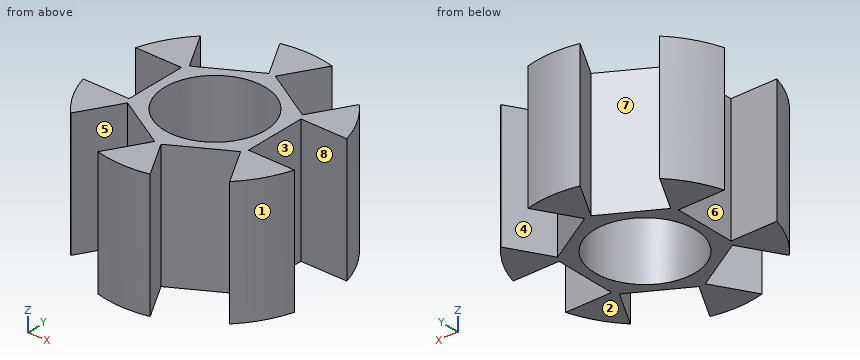
from build123d import *

# Parameters (mm, degrees)
SKETCH1_R           = 8.75
SKETCH1_R_2         = 4
BOSS_EXTRUDE1_DEPTH = 5
SKETCH2_W           = 4.9
SKETCH2_H           = 10
CUT_EXTRUDE3_DEPTH  = 4
CIRPATTERN1_COUNT   = 6


with BuildPart() as part:
    # Sketch1 → Boss-Extrude1 (new body, symmetric)
    with BuildSketch(Plane.XY):
        Circle(SKETCH1_R)
        Circle(SKETCH1_R_2, mode=Mode.SUBTRACT)
    extrude(amount=BOSS_EXTRUDE1_DEPTH, both=True)

    # Sketch2 → Cut-Extrude3 (cut)
    with BuildSketch(Plane(origin=(-8.75, -17.193061184, 0), x_dir=(0, -1, 0), z_dir=(1, 0, 0))):
        with Locations((-17.193061184, 0)):
            Rectangle(SKETCH2_W, SKETCH2_H)
    cut_extrude3 = extrude(amount=CUT_EXTRUDE3_DEPTH, mode=Mode.SUBTRACT)

    # CirPattern1: Cut-Extrude3 ×6 about axis
    cirpattern1_axis = Axis((0, 0, 0), (0, 0, 1))
    for i in range(1, CIRPATTERN1_COUNT):
        add(cut_extrude3.rotate(cirpattern1_axis, i * 360 / CIRPATTERN1_COUNT), mode=Mode.SUBTRACT)


solid = part.part
CAD build for the part. Positions are in the model's coordinates, mm. Face numbers are marked on the shaded views. A direction names the side the tool comes from. Give positions to 0.01 mm unless a question says otherwise; leave off trailing zeros. Write each loop counter-clockwise with the first axis right and the second up, starting at its lowest first coordinate (ties: lowest second). Pieces come first, ordered by that corner, then holes. Notation, with made-up numbers: (69, -35) - (92, -35) arc R20 cw to (92, -7) - close; hole circle Ø6 at (-13.75, 66). An arc over 180 degrees is marked (long way). Answer as CSV lines item,"result".
Q1. 3-axis set-ups, long thin cutter, end or side, ignore diameter. For the marked faces 4, 5, 6, 7 and 8: which of +Z, -Z, +X, -X, +Y, -Y reach the whole face in a straight line?
Result set:
face 4,"+Z, -Z, +Y"
face 5,"+Z, -Z, -Y"
face 6,"+Z, -Z, -X"
face 7,"+Z, -Z"
face 8,"+Z, -Z, +X"
Q2. Band-saw the part on D-D (x = -4.25). Give the cut face in (y, z), and give its area (3 significant figures).
Result set:
outline,"(-3.03, -5) - (3.03, -5) - (3.03, 5) - (-3.03, 5) - close"
area,"60.6 mm²"
Q3. Band-saw the part on A-A (x = 0). Give the cut face in (y, z).
Result set:
outline,"(-8.75, -5) - (-4, -5) - (-4, 5) - (-8.75, 5) - close; (4, -5) - (8.75, -5) - (8.75, 5) - (4, 5) - close"
Q4. Pull direction Y, two halves, no side cores. Call the marked faces 1, 2 and 3: released by +Y, released by -Y, zero draft, split by the parting line, or undercut.
Result set:
face 1,"released by -Y"
face 2,"zero draft"
face 3,"undercut"
Q5. Band-saw the part on B-B (y = 0). Give the cut face in (x, z).
Result set:
outline,"(-4.75, -5) - (-4, -5) - (-4, 5) - (-4.75, 5) - close; (4, -5) - (4.75, -5) - (4.75, 5) - (4, 5) - close"
Q6. Drill centre lines: line 1 (Y direction, x = 0, z = -2.5); line 2 (X direction, y = -4.5, z = 2.75); line 3 (Y direction, x = -0.5, z = 2.75). Where is each one in solid material? Low to high. Write a range as from..to.
Result set:
line 1,"-8.75..-4, 4..8.75"
line 2,"-7.5..-5.43, -1.71..1.71, 5.43..7.5"
line 3,"-8.74..-5.77, -5.2..-3.97, 3.97..5.2, 5.77..8.74"
Q7. Band-saw the part on C-C (z = 3.5). Give the cut face in (x, y), and give its area (3 significant figures).
Result set:
outline,"(-8.4, -2.45) arc R8.75 ccw to (-6.32, -6.05) - (-4.5, -2.89) - (-0.25, -5.34) - (-2.08, -8.5) arc R8.75 ccw to (2.08, -8.5) - (0.25, -5.34) - (4.5, -2.89) - (6.32, -6.05) arc R8.75 ccw to (8.4, -2.45) - (4.75, -2.45) - (4.75, 2.45) - (8.4, 2.45) arc R8.75 ccw to (6.32, 6.05) - (4.5, 2.89) - (0.25, 5.34) - (2.08, 8.5) arc R8.75 ccw to (-2.08, 8.5) - (-0.25, 5.34) - (-4.5, 2.89) - (-6.32, 6.05) arc R8.75 ccw to (-8.4, 2.45) - (-4.75, 2.45) - (-4.75, -2.45) - close; hole circle Ø8 at (0, 0)"
area,"76.1 mm²"
Q8. Flat gauge pins, fed straight in: pin 1 Ø1.5 at (y, z) = (-1, 0.5) entering from -X; pin 2 Ø1 at (x, z) = (1, -1.5) entering from -Y; pin 3 Ø4 at (y, z) = (-0.5, 0.5) entering from +X; pin 4 Ø4 at (x, z) = (6.5, 1.5) entering from -Y. Where does each tip first touch, or does it go through?
Result set:
pin 1,"x = -4.75"
pin 2,"y = -8.74"
pin 3,"x = 8.4"
pin 4,"y = -6.05"
